The listing builds one solid part. Answer for the finished solid, in the listing's coordinates (mm). Face numbers are marked on the shaded views. A direction names the side the tool comes from. Round coordinates to 2 decimals unless told otherwise and drop trailing zeros. Order: outer loops, then holes, each group sorted by start corner. A loop starts at its lowest first (then second) coordinate and runs counter-clockwise, first axis right, second up. Notation, with made-up numbers: M 76.5,29 L 92.5,29 A29 ccw 92.5,52 Z; hole C -32.75,15 d4. An arc over 180 degrees is marked long. Put each result on its own line as item: value. Start each with the question number.
1. The mould has two halves that part along Z. Classify the marked faces 4, 5 and 6: +Z half, -Z half, draft (parallel to the pull), parting line (faces both ways), or undercut.
2. The part is cut by section C-C (z = -6.5). Give the vertices of the cut face in (x, y).
3. Each of these flat-tipped pins is pushed along its axis until it touches: pin 1 Ø6 at (y, z) = (116.5, 10.5) entering from -X; pin 2 Ø1.6 at (y, z) = (89, -12) entering from +X; pin 3 Ø4 at (y, z) = (89.5, -1) entering from +X. Where does it stop, or does it pass through?
4. The part is cut by section B-B (x = 13.5). Give the vertices of the cut face in (y, z), then the cut area to 3 significant figures.
5. Consider line 1 (Z direction, x = 34.5, y = 103); line 2 (Z direction, x = 27, y = 114.5); line 3 (Y direction, x = 13, z = 5.5). Determine where each line is inside the solid, lowest interval first.
6. The part is cut by section A-A (y = 113.5). Give the vertices of the cut face in (x, z).
7. Which of the six approach directions +Z, -Z, +X, -X, +Y, -Y give full straight-line access (tool end or side, diameter ignored) to the marked faces 1, 2 and 3?
8. The part is cut by section D-D (y = 98). Give the vertices of the cut face in (x, z), then the cut area to 3 significant figures.
from build123d import *

# Parameters (mm, degrees)
EXTRUDE_1_DEPTH     = 5
EXTRUDE_1_2_DEPTH   = 5
EXTRUDE_1_3_DEPTH   = 5
EXTRUDE_2_DEPTH     = 13
EXTRUDE_3_DEPTH     = 0.75
CUT_EXTRUDE_1_DEPTH = 6
CUT_EXTRUDE_2_DEPTH = 4
EXTRUDE_5_DEPTH     = 4
CHAMFER_1_SIZE      = 1


with BuildPart() as part:
    # Sketch 1 → Extrude 1 (new body)
    with BuildSketch(Plane.XY):
        Polygon((21.49998914, 95.432607267), (27.49998914, 89.432607267), (29.49998914, 87.432607267), (31.99998914, 84.932607267), (32.707095921, 85.639714048), (30.914202702, 87.432607267), (30.207095921, 88.139714048), (31.689328968, 89.621947095), (33.103542531, 88.207733533), (35.224862874, 90.329053877), (33.810649312, 91.743267439), (35.292882359, 93.225500486), (35.99998914, 92.518393705), (37.792882359, 90.725500486), (38.49998914, 91.432607267), (35.99998914, 93.932607267), (33.99998914, 95.932607267), (27.99998914, 101.932607267), (27.99998914, 95.432607267), align=None)
    extrude(amount=EXTRUDE_1_DEPTH)



with BuildPart() as body_2:
    # Sketch 1 → Extrude 1 2 (new body)
    with BuildSketch(Plane.XY):
        Polygon((5.99998914, 87.432607267), (5.99998914, 95.432607267), (0.99998914, 95.432607267), (-1.086e-05, 94.432607267), (-1.086e-05, 88.432607267), (0.99998914, 87.432607267), (3.49998914, 84.932607267), (4.207095921, 85.639714048), (2.414202702, 87.432607267), (1.707095921, 88.139714048), (2.767756093, 89.20037422), (4.535523046, 87.432607267), align=None)
    extrude(amount=EXTRUDE_1_2_DEPTH)


with BuildPart() as body_3:
    # Sketch 1 → Extrude 1 3 (new body)
    with BuildSketch(Plane.XY):
        Polygon((27.99998914, 117.432607267), (35.99998914, 117.432607267), (35.99998914, 118.897073361), (34.232222187, 120.664840314), (35.292882359, 121.725500486), (35.99998914, 121.018393705), (37.792882359, 119.225500486), (38.49998914, 119.932607267), (35.99998914, 122.432607267), (34.99998914, 123.432607267), (28.99998914, 123.432607267), (27.99998914, 122.432607267), align=None)
    extrude(amount=EXTRUDE_1_3_DEPTH)


with BuildPart() as part_1:
    add(part.part)

    add(body_2.part)  # Extrude 2 merges body 2

    add(body_3.part)  # Extrude 2 merges body 3
    # Sketch 2 → Extrude 2 (add)
    with BuildSketch(Plane.XY.offset(5)):
        Polygon((34.99998914, 123.432607267), (28.99998914, 123.432607267), (27.99998914, 122.432607267), (27.99998914, 95.432607267), (0.99998914, 95.432607267), (-1.086e-05, 94.432607267), (-1.086e-05, 88.432607267), (0.99998914, 87.432607267), (35.99998914, 87.432607267), (35.99998914, 122.432607267), align=None)
    extrude(amount=EXTRUDE_2_DEPTH)

    # Sketch 3 → Extrude 3 (add)
    with BuildSketch(Plane(origin=(0, 0, 5), x_dir=(-1, 0, 0), z_dir=(0, 0, -1))):
        Polygon((-27.99998914, 117.432607267), (-35.99998914, 117.432607267), (-35.99998914, 93.932607267), (-27.99998914, 101.932607267), align=None)
    extrude_3 = extrude(amount=EXTRUDE_3_DEPTH)

    # Mirror 1: Extrude 3 across plane
    add(extrude_3.mirror(Plane(origin=(61.716298204, 61.716298204, 0), x_dir=(0, 0, 1), z_dir=(-0.707106781, -0.707106781, 0))))

    # Sketch 4 → Cut-Extrude 1 (cut)
    with BuildSketch(Plane.XY.offset(14)):
        Polygon((33.99998914, 114.432607267), (35.99998914, 114.432607267), (35.99998914, 93.932607267), (33.99998914, 95.932607267), align=None)
    cut_extrude_1 = extrude(amount=-CUT_EXTRUDE_1_DEPTH, mode=Mode.SUBTRACT)

    # Sketch 6 → Cut-Extrude 2 (cut)
    with BuildSketch(Plane.XY.offset(14)):
        Polygon((31.99998914, 123.432607267), (34.99998914, 123.432607267), (35.99998914, 122.432607267), (35.99998914, 117.72001524), align=None)
    cut_extrude_2 = extrude(amount=-CUT_EXTRUDE_2_DEPTH, mode=Mode.SUBTRACT)

    # Mirror 2: Cut-Extrude 1, Cut-Extrude 2 across plane
    add(cut_extrude_1.mirror(Plane(origin=(61.716298204, 61.716298204, 0), x_dir=(0, 0, 1), z_dir=(-0.707106781, -0.707106781, 0))), mode=Mode.SUBTRACT)
    add(cut_extrude_2.mirror(Plane(origin=(61.716298204, 61.716298204, 0), x_dir=(0, 0, 1), z_dir=(-0.707106781, -0.707106781, 0))), mode=Mode.SUBTRACT)

    # Sketch 7 → Extrude 5 (add)
    with BuildSketch(Plane.XY.offset(18)):
        Polygon((0.99998914, 95.432607267), (27.99998914, 95.432607267), (27.99998914, 122.432607267), align=None)
    extrude(amount=-EXTRUDE_5_DEPTH)

    # Mirror 4: part across plane


with BuildPart() as part_2:
    add(part_1.part)
    add(part_1.part.mirror(Plane(origin=(0, 0, 0), x_dir=(1, 0, 0), z_dir=(0, 0, -1))))

    # Chamfer 1
    chamfer_1_edges = [part_2.edges().sort_by_distance(p)[0] for p in [
        (35.99998914, 87.432607267, -11.5),
        (35.99998914, 87.432607267, 11.5),
    ]]
    chamfer(chamfer_1_edges, length=CHAMFER_1_SIZE)


solid = part_2.part
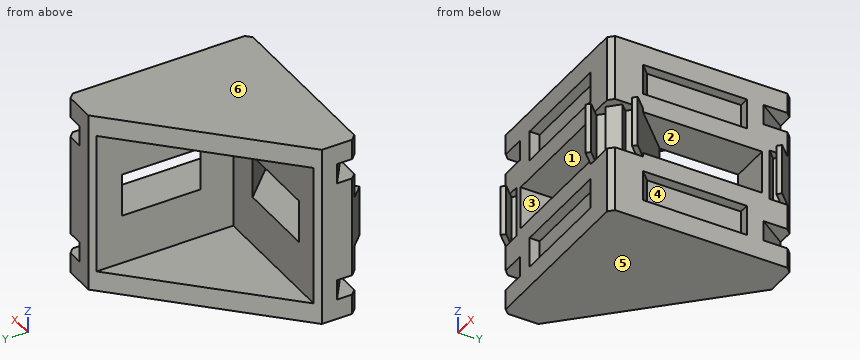
Resolved:
1. face 4: undercut
1. face 5: -Z half
1. face 6: +Z half
2. outline: M 0,88.43 L 1,87.43 L 35,87.43 L 36,88.43 L 36,122.43 L 35,123.43 L 29,123.43 L 28,122.43 L 28,95.43 L 1,95.43 L 0,94.43 Z
3. pin 1: x = 28
3. pin 2: x = 36
3. pin 3: x = 38.5
4. outline: M 87.43,-18 L 107.93,-18 L 107.93,-14 L 95.43,-14 L 95.43,-4.25 L 87.43,-4.25 L 87.43,-8 L 89.43,-8 L 89.43,-14 L 87.43,-14 Z; M 87.43,4.25 L 95.43,4.25 L 95.43,14 L 107.93,14 L 107.93,18 L 87.43,18 L 87.43,14 L 89.43,14 L 89.43,8 L 87.43,8 Z
4. area: 296 mm2
5. line 1: -18 to -14, -8 to -4.25, 4.25 to 8, 14 to 18
5. line 2: -18 to -14, 14 to 18
5. line 3: 87.43 to 95.43
6. outline: M 19.07,-18 L 36,-18 L 36,-14 L 34,-14 L 34,-8 L 36,-8 L 36,-4.25 L 28,-4.25 L 28,-14 L 19.07,-14 Z; M 19.07,14 L 28,14 L 28,4.25 L 36,4.25 L 36,8 L 34,8 L 34,14 L 36,14 L 36,18 L 19.07,18 Z
7. face 1: -Y
7. face 2: +X
7. face 3: +Y, -Y
8. outline: M 3.57,-18 L 36,-18 L 36,-14 L 34,-14 L 34,-8 L 36,-8 L 36,-4.25 L 31.93,-4.25 L 31.93,4.25 L 36,4.25 L 36,8 L 34,8 L 34,14 L 36,14 L 36,18 L 3.57,18 L 3.57,14 L 28,14 L 28,-14 L 3.57,-14 Z
8. area: 425 mm2
